from build123d import *

# Parameters (mm, degrees)
SKETCH1_R           = 1.65
SKETCH1_R_2         = 5
BOSS_EXTRUDE1_DEPTH = 3


with BuildPart() as part:
    # Sketch1 → Boss-Extrude1 (new body)
    with BuildSketch(Plane.XY):
        with BuildLine():
            Line((16.563434593, 11.720833187), (6.963921749, 2.121320344))
            ThreePointArc((6.963921749, 2.121320344), (6.085242093, 0), (6.963921749, -2.121320344))
            Line((6.963921749, -2.121320344), (16.563434593, -11.720833187))
            ThreePointArc((16.563434593, -11.720833187), (16.563434593, -16.563434593), (11.720833187, -16.563434593))
            Line((11.720833187, -16.563434593), (2.121320344, -6.963921749))
            ThreePointArc((2.121320344, -6.963921749), (0, -6.085242093), (-2.121320344, -6.963921749))
            Line((-2.121320344, -6.963921749), (-11.720833187, -16.563434593))
            ThreePointArc((-11.720833187, -16.563434593), (-16.56343546, -16.563437193), (-16.563436326, -11.720834921))
            Line((-16.563436326, -11.720834921), (-6.963921749, -2.121320344))
            ThreePointArc((-6.963921749, -2.121320344), (-6.085242093, 0), (-6.963921749, 2.121320344))
            Line((-6.963921749, 2.121320344), (-16.563434593, 11.720833187))
            ThreePointArc((-16.563434593, 11.720833187), (-16.563434593, 16.563434593), (-11.720833187, 16.563434593))
            Line((-11.720833187, 16.563434593), (-2.121320344, 6.963921749))
            ThreePointArc((-2.121320344, 6.963921749), (0, 6.085242093), (2.121320344, 6.963921749))
            Line((2.121320344, 6.963921749), (11.720833187, 16.563434593))
            ThreePointArc((11.720833187, 16.563434593), (16.563436326, 16.563436326), (16.563434593, 11.720833187))
        make_face()
        with Locations((-14.14213389, 14.14213389)):
            Circle(SKETCH1_R, mode=Mode.SUBTRACT)
        with Locations((14.142135624, 14.142135624)):
            Circle(SKETCH1_R, mode=Mode.SUBTRACT)
        with Locations((-14.142135624, -14.142135624)):
            Circle(SKETCH1_R, mode=Mode.SUBTRACT)
        with Locations((14.14213389, -14.14213389)):
            Circle(SKETCH1_R, mode=Mode.SUBTRACT)
        Circle(SKETCH1_R_2, mode=Mode.SUBTRACT)
        with Locations((-6.759874347, 6.759874347)):
            Circle(SKETCH1_R, mode=Mode.SUBTRACT)
        with Locations(Location((6.759874347, 6.759874347, 0), (0, 0, 180))):
            Circle(SKETCH1_R, mode=Mode.SUBTRACT)
        with Locations((6.759874347, -6.759874347)):
            Circle(SKETCH1_R, mode=Mode.SUBTRACT)
        with Locations(Location((-6.759874347, -6.759874347, 0), (0, 0, 180))):
            Circle(SKETCH1_R, mode=Mode.SUBTRACT)
    extrude(amount=BOSS_EXTRUDE1_DEPTH)


solid = part.part
Model file for the job. Use its own axes, mm. A direction names the side the tool comes from. Give positions to 0.01 mm unless a question says otherwise; leave off trailing zeros. Loops run counter-clockwise (first coordinate to the right, second up) from the corner with the lowest first, then second, coordinate; pieces in that order, holes last. Notation, with made-up numbers: (32.25, 22) -> (73.25, 22) arc R32 cw to (73.25, 57) -> close; hole circle Ø8 at (-11, 9.5). An arc over 180 degrees is marked (long way). Use a Markdown table: item, result. Add a question column.
(1) Tool access for faces 1 (the cylindrical face through (12.8, -15.1, 1.5)), 2 (the flat face through (11.696, -6.854, 1.479)), 3 (the flat face through (6.99, -11.83, 1.48)), 4 (the flat face through (-11.83, -6.99, 1.48)), 5 (the flat face through (-6.99, 11.83, 1.48)): list every direction of +Z, -Z, +X, -X, +Y, -Y with a clear straight run to the whole face (end or side of a thin tool).
(2) Slice it at C-C on y = -7.5. List the corners of the cut face in (x, z), and give its area (3 significant figures).
(3) Drop a flat-ended pin along its axis: pin 1 Ø2 at (x, y) = (6.76, -6.76) entering from -Z. Give the stop position or say it passes through.
(4) Slice it at A-A on y = 0. List the corners of the cut face in (x, z).
(5) Mould opens along X. For faces 6 (the flat face through (-11.696, 6.854, 1.479)), 7 (the flat face through (11.83, 6.99, 1.48)), 8 (the cylindrical face through (-0.033, 6.085, 1.479)) say: +X half, -X half, draft (parallel to the pull), parting line (faces both ways), or undercut.
(6) Slice it at D-D on x = 6.5. List the corners of the cut face in (y, z).
(7) Wall check: line 1 along X through (y, z) = (-13.5, 0.3); line 2 along Y through (x, z) = (0, 0.85); line 3 along Y through (x, z) = (-7.5, 2.55). Give the ranges that are in metal, low to high.
Filled sheet:
| question | item | result |
|---|---|---|
| 1 | face 1 | +Z, -Z |
| 1 | face 2 | +Z, -Z, +X |
| 1 | face 3 | +Z, -Z, -Y |
| 1 | face 4 | +Z, -Z, -X |
| 1 | face 5 | +Z, -Z, +Y |
| 2 | outline | (-12.34, 0) -> (-8.23, 0) -> (-8.23, 3) -> (-12.34, 3) -> close; (-5.29, 0) -> (-2.66, 0) -> (-2.66, 3) -> (-5.29, 3) -> close; (2.66, 0) -> (5.29, 0) -> (5.29, 3) -> (2.66, 3) -> close; (8.23, 0) -> (12.34, 0) -> (12.34, 3) -> (8.23, 3) -> close |
| 2 | area | 40.4 mm2 |
| 3 | pin 1 | through |
| 4 | outline | (-6.09, 0) -> (-5, 0) -> (-5, 3) -> (-6.09, 3) -> close; (5, 0) -> (6.09, 0) -> (6.09, 3) -> (5, 3) -> close |
| 5 | face 6 | -X half |
| 5 | face 7 | +X half |
| 5 | face 8 | undercut |
| 6 | outline | (-11.34, 0) -> (-8.39, 0) -> (-8.39, 3) -> (-11.34, 3) -> close; (-5.13, 0) -> (-1.52, 0) -> (-1.52, 3) -> (-5.13, 3) -> close; (1.52, 0) -> (5.13, 0) -> (5.13, 3) -> (1.52, 3) -> close; (8.39, 0) -> (11.34, 0) -> (11.34, 3) -> (8.39, 3) -> close |
| 7 | line 1 | -17.51 to -15.66, -12.62 to -8.66, 8.66 to 12.62, 15.66 to 17.51 |
| 7 | line 2 | -6.09 to -5, 5 to 6.09 |
| 7 | line 3 | -12.34 to -8.23, -5.29 to -2.66, 2.66 to 5.29, 8.23 to 12.34 |
